from build123d import *

# Parameters (mm, degrees)
SKETCH1_R                                        = 19.25
SKETCH1_R_2                                      = 16.25
BOSS_EXTRUDE1_DEPTH                              = 5
BOSS_EXTRUDE2_DEPTH                              = 8
CBORE_FOR_1_4_SOCKET_HEAD_CAP_SCREW2_D           = 6.7564
CBORE_FOR_1_4_SOCKET_HEAD_CAP_SCREW2_CBORE_D     = 11.1125
CBORE_FOR_1_4_SOCKET_HEAD_CAP_SCREW2_CBORE_DEPTH = 6.35
FILLET1_R                                        = 10


with BuildPart() as part:
    # Sketch1 → Boss-Extrude1 (new body)
    with BuildSketch(Plane(origin=(0, 0, 0), x_dir=(1, 0, 0), z_dir=(0, 1, 0))):
        with Locations(Location((0, 0, 0), (0, 0, 270))):
            Circle(SKETCH1_R)
        with Locations(Location((0, 0, 0), (0, 0, 270))):
            Circle(SKETCH1_R_2, mode=Mode.SUBTRACT)
    extrude(amount=BOSS_EXTRUDE1_DEPTH)

    # Sketch2 → Boss-Extrude2 (add)
    with BuildSketch(Plane(origin=(0, 0, 0), x_dir=(1, 0, 0), z_dir=(0, 1, 0))):
        with BuildLine():
            Line((-6.35, -31.75), (31.75, -31.75))
            Line((31.75, -31.75), (31.75, 6.35))
            Line((31.75, 6.35), (18.172506707, 6.35))
            ThreePointArc((18.172506707, 6.35), (18.978715105, 3.220383975), (19.25, 0))
            ThreePointArc((19.25, 0), (11.142822802, -15.697133496), (-6.35, -18.172506707))
            Line((-6.35, -18.172506707), (-6.35, -31.75))
        make_face()
    extrude(amount=BOSS_EXTRUDE2_DEPTH)

    # CBORE for 1/4 Socket Head Cap Screw2 (through all)
    with Locations(Plane(origin=(0, 8, 0), x_dir=(1, 0, 0), z_dir=(0, 1, 0))):
        with Locations((0, -25.4), (25.4, -25.4), (25.4, 0)):
            CounterBoreHole(CBORE_FOR_1_4_SOCKET_HEAD_CAP_SCREW2_D / 2, CBORE_FOR_1_4_SOCKET_HEAD_CAP_SCREW2_CBORE_D / 2, CBORE_FOR_1_4_SOCKET_HEAD_CAP_SCREW2_CBORE_DEPTH)

    # Fillet1
    # the kernel refuses this fillet: 10 mm, written as the material it adds along each edge
    with BuildSketch(Plane(origin=(18.172506707, 0, -6.35), x_dir=(-0.4481163543899531, 0, -0.8939752417870743), z_dir=(0, 1, 0))) as fillet1_piece_1:
        with BuildLine():
            CenterArc((6.21468839, -9.917563599), FILLET1_R, 97.362002187, 56.015102529)
            Line((-2.725064028, -5.436400055), (0, 0))
            ThreePointArc((0, 0), (2.46665467, -0.158690073), (4.93330934, 0))
        make_face()
    extrude(amount=5)
    with BuildSketch(Plane(origin=(-6.35, 0, 18.172506707), x_dir=(-0.8939752417870848, 0, -0.44811635438993225), z_dir=(0, 1, 0))) as fillet1_piece_2:
        with BuildLine():
            CenterArc((6.21468839, 9.917563599), FILLET1_R, 206.622895283, 56.015102529)
            Line((-2.725064028, 5.436400055), (0, 0))
            ThreePointArc((0, 0), (2.46665467, 0.158690073), (4.93330934, 0))
        make_face()
    extrude(amount=5)
    # the kernel refuses this fillet: 10 mm, written as the material it takes off along each edge
    with BuildSketch(Plane(origin=(0, 8, 0), x_dir=(-0.9534219544060213, 0, 0.3016398131159126), z_dir=(-0.3016398131159126, 0, -0.9534219544060213))) as fillet1_2_piece_1:
        with BuildLine():
            CenterArc((26.391428429, -10), FILLET1_R, 90, 45.572995999)
            Line((26.391428429, 0), (19.25, 0))
            Line((19.25, 0), (19.25, -3))
        make_face()
    revolve(axis=Axis((0, 8, 0), (0, 1, 0)), revolution_arc=234.887758498, mode=Mode.SUBTRACT)


solid = part.part
Geometry check sheet. Reference: the model listing, model coordinates, mm. A direction names the side the tool comes from. Coordinates: 2 decimals unless noted, no trailing zeros. Order: outer loops, then holes, each group sorted by start corner. A loop starts at its lowest first (then second) coordinate and runs counter-clockwise, first axis right, second up. Notation, with made-up numbers: (89.5, 58) -> (110.5, 58) arc R19 cw to (110.5, 93) -> close; hole circle Ø3 at (-7, 23.25). An arc over 180 degrees is marked (long way). Use a Markdown table: item, result. Add a question column.
1. Cross-section at D-D (x = 0). Enter the section's corners in (y, z), and give its area (3 significant figures).
2. Mould release check, pull along Z, two halves, no side actions. Record for faces 6 (the face through (31.75, 4, 13)), 7 (the face through (28, 1.65, 28)), 8 (the face through (12, 4, 31.75)), 9 (the face through (19.5, 2.46, -7.55)): pulls with the +Z half, pulls with the -Z half, needs draft (parallel to the pull), parting line crosses it, or undercut.
3. Go/stop test with flat-tipped pins: pin 1 Ø5.5 at (x, z) = (23.5, 2.5) entering from +Y; pin 2 Ø3.5 at (x, z) = (25, 26) entering from +Y; pin 3 Ø10 at (x, z) = (25.4, 25.4) entering from +Y; pin 4 Ø13 at (x, z) = (10, -1.5) entering from +Y. Record where each tip stops, or that it passes through.
4. Cross-section at B-B (x = -7). Enter the section's corners in (y, z) (3 decimals), and give its area (3 significant figures).
5. Set-up check for faces 1 (the face through (27, 4, -6.35)), 2 (the face through (30.53, 4.87, 2.13)), 3 (the face through (-7.5, 2.5, 19.6)), 4 (the face through (-6.35, 4, 26)), 5 (the face through (0.73, 0.81, 28.7)): record each of +Z, -Z, +X, -X, +Y, -Y from which the full face is reachable in a straight line by a thin tool's end or side.
6. Cross-section at C-C (z = 0). Enter the section's corners in (x, y).
7. Cross-section at A-A (z = -15.5). Enter the section's corners in (x, y).
8. Material ranges on L1, parallel to Z at x = 25.4, y = 0.9; L2, parallel to X at y = 4.25, z = 25.4, recorded low to high.
Filled sheet:
| question | item | result |
|---|---|---|
| 1 | outline | (0, -19.25) -> (5, -19.25) -> (5, -16.25) -> (0, -16.25) -> close; (0, 16.25) -> (5, 16.25) -> (5, 19.25) arc R10 ccw to (5.56, 19.84) -> (1.65, 19.84) -> (1.65, 22.02) -> (0, 22.02) -> close; (0, 28.78) -> (1.65, 28.78) -> (1.65, 30.96) -> (8, 30.96) -> (8, 31.75) -> (0, 31.75) -> close |
| 1 | area | 46.7 mm2 |
| 2 | face 6 | needs draft |
| 2 | face 7 | undercut |
| 2 | face 8 | pulls with the +Z half |
| 2 | face 9 | pulls with the -Z half |
| 3 | pin 1 | y = 7.75 |
| 3 | pin 2 | through |
| 3 | pin 3 | y = 1.65 |
| 3 | pin 4 | y = 5 |
| 4 | outline | (0, -17.932) -> (5, -17.932) -> (5, -14.665) -> (0, -14.665) -> close; (0, 14.665) -> (5, 14.665) -> (5, 20.707) -> (0, 20.707) -> close |
| 4 | area | 46.5 mm2 |
| 5 | face 1 | -Z, +X, +Y |
| 5 | face 2 | +Y |
| 5 | face 3 | +Z, -X, +Y, -Y |
| 5 | face 4 | +Z, -X, +Y |
| 5 | face 5 | +Y, -Y |
| 6 | outline | (-19.25, 0) -> (-16.25, 0) -> (-16.25, 5) -> (-19.25, 5) -> close; (16.25, 0) -> (22.02, 0) -> (22.02, 1.65) -> (19.84, 1.65) -> (19.84, 5.56) arc R10 ccw to (19.25, 5) -> (16.25, 5) -> close; (28.78, 0) -> (31.75, 0) -> (31.75, 8) -> (30.96, 8) -> (30.96, 1.65) -> (28.78, 1.65) -> close |
| 7 | outline | (-11.42, 0) -> (-4.88, 0) -> (-4.88, 5) -> (-11.42, 5) -> close; (4.88, 0) -> (11.42, 0) -> (11.42, 5) -> (4.88, 5) -> close |
| 8 | L1 | -6.35 to -3.38, 3.38 to 22.02, 28.78 to 31.75 |
| 8 | L2 | -6.35 to -5.56, 5.56 to 19.84, 30.96 to 31.75 |
